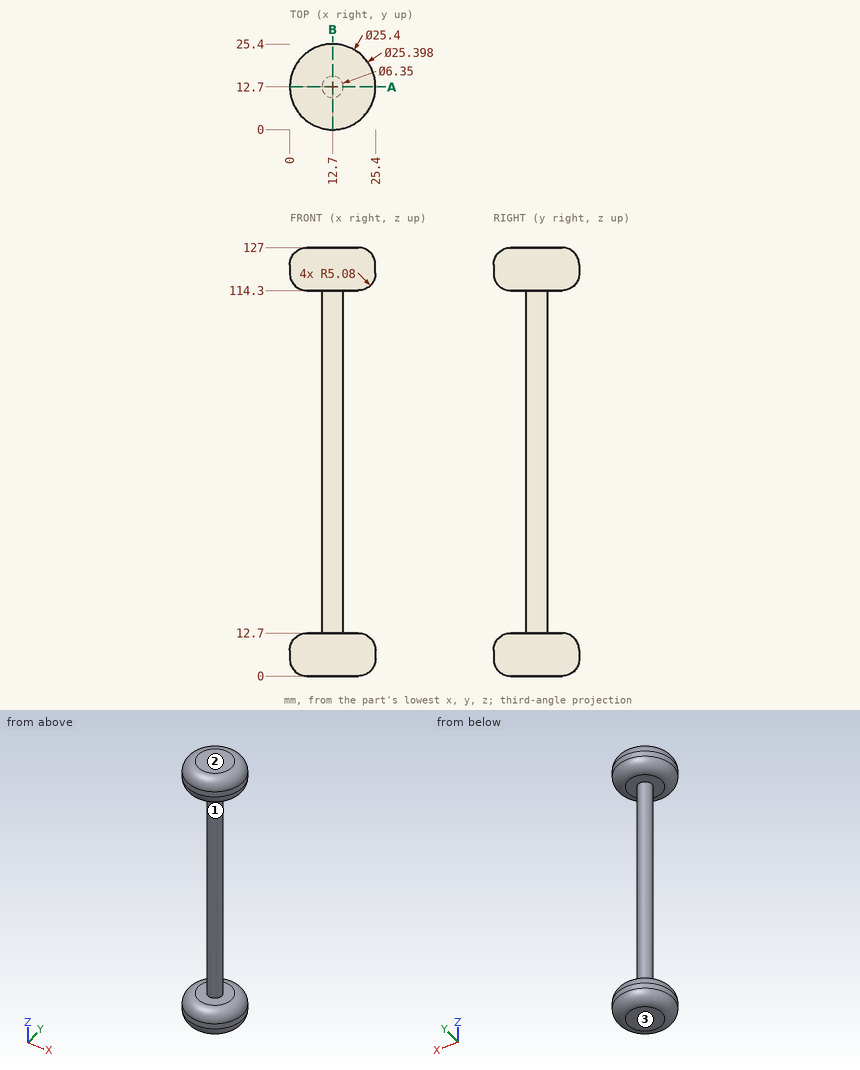
Here's the drawing with two shaded views (mm, measured from the low corner). I have some questions. Coordinates: 2 decimals unless noted, no trailing zeros. Loops run counter-clockwise (first coordinate to the right, second up) from the corner with the lowest first, then second, coordinate; pieces in that order, holes last. Notation, with made-up numbers: M 21,64.25 L 36,64.25 A9 cw 36,71.25 Z; hole C -21.75,-32.5 d1. An arc over 180 degrees is marked long. Put each result on its own line as item: value. Start each with the question number.
(1) I need wall thicknesses on probe 1 along Z at (x, y) = (8.5, 17.25); probe 2 along Z at (x, y) = (2.75, 11) (1 decimal); probe 3 along X at (y, z) = (12.25, 44.5). Which ranges of each line are inside material? Lowest first, please.
(2) We'd pull the mould along Z, two halves only. Please class the marked faces 1, 2 and 3: +Z half, -Z half, draft (parallel to the pull), parting line (faces both ways), or undercut.
(3) Will these pins go through, and if not, where does the flat tip stop? pin 1 Ø12 at (x, z) = (20, 86.5) entering from -Y; pin 2 Ø6 at (x, z) = (11.5, 72) entering from +Y (3 decimals); pin 3 Ø12 at (x, z) = (5.5, 74) entering from +Y.
(4) Imagine slicing it at A-A on y = 12.7. List the corners of the cut face in (x, z) for me (1 decimal), and give its area (3 significant figures).
Worked answers:
1. probe 1: z = 0 to 12.7, 114.3 to 127
1. probe 2: z = 0.6 to 12.1, 114.9 to 126.4
1. probe 3: x = 9.56 to 15.84
2. face 1: undercut
2. face 2: +Z half
2. face 3: -Z half
3. pin 1: stops at y = 9.8
3. pin 2: stops at y = 15.875
3. pin 3: stops at y = 15.64
4. outline: M 0,5.1 A5.1 ccw 5.1,0 L 20.3,0 A5.1 ccw 25.4,5.1 L 25.4,7.6 A5.1 ccw 20.3,12.7 L 15.9,12.7 L 15.9,114.3 L 20.3,114.3 A5.1 ccw 25.4,119.4 L 25.4,121.9 A5.1 ccw 20.3,127 L 5.1,127 A5.1 ccw 0,121.9 L 0,119.4 A5.1 ccw 5.1,114.3 L 9.5,114.3 L 9.5,12.7 L 5.1,12.7 A5.1 ccw 0,7.6 Z
4. area: 1,250 mm2
